Source: CAD feature listing. Evaluate the final solid. Frame: model axes, mm. Face numbers are marked on the shaded views. A direction names the side the tool comes from. Give positions to 0.01 mm unless a question says otherwise; leave off trailing zeros. Order: outer loops, then holes, each group sorted by start corner. A loop starts at its lowest first (then second) coordinate and runs counter-clockwise, first axis right, second up. Notation, with made-up numbers: (5.25, 23) - (11.25, 23) arc R19 ccw to (11.25, 32) - close; hole circle Ø11 at (39.5, 48.5). An arc over 180 degrees is marked (long way). Answer as CSV lines item,"result".
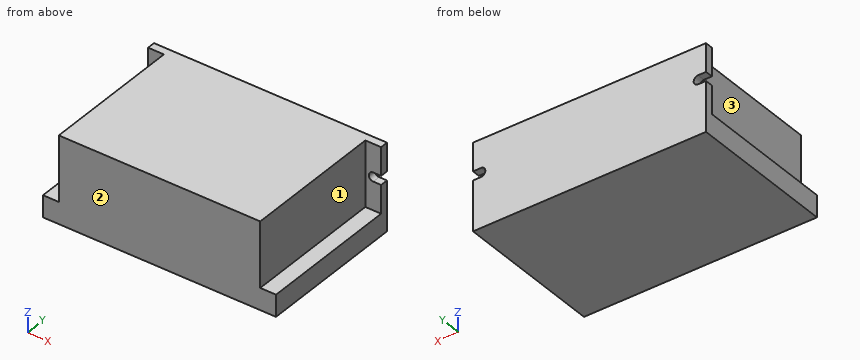
```python
from build123d import *

# Parameters (mm, degrees)
ESQUISSE1_W             = 118
ESQUISSE1_H             = 75.5
BOSS_EXTRU_1_DEPTH      = 11
BOSS_EXTRU_2_DEPTH      = 33
ENL_V_MAT_EXTRU_1_REACH = 107.929


with BuildPart() as part:
    # Esquisse1 → Boss.-Extru.1 (new body)
    with BuildSketch(Plane.XY):
        with Locations((-5.596837945, -6.384387352)):
            Rectangle(ESQUISSE1_W, ESQUISSE1_H)
    extrude(amount=BOSS_EXTRU_1_DEPTH)

    # Esquisse2 → Boss.-Extru.2 (add)
    with BuildSketch(Plane.XY.offset(11)):
        Polygon((-64.596837945, 31.365612648), (53.403162055, 31.365612648), (53.403162055, 27.365612648), (45.403162055, 27.365612648), (45.403162055, -44.134387352), (-56.596837945, -44.134387352), (-56.596837945, 27.365612648), (-64.596837945, 27.365612648), align=None)
    extrude(amount=BOSS_EXTRU_2_DEPTH)

    # Esquisse3 → Enlèv. mat.-Extru.1 (cut, up to next)
    with BuildSketch(Plane.XZ.offset(-27.365612648), mode=Mode.PRIVATE) as enl_v_mat_extru_1_sk1:
        with BuildLine():
            Line((-64.596837945, 29.75), (-60.596837945, 29.75))
            ThreePointArc((-60.596837945, 29.75), (-58.346837945, 27.5), (-60.596837945, 25.25))
            Line((-60.596837945, 25.25), (-64.596837945, 25.25))
            Line((-64.596837945, 25.25), (-64.596837945, 29.75))
        make_face()
    enl_v_mat_extru_1_tool1 = extrude(enl_v_mat_extru_1_sk1.sketch, amount=-ENL_V_MAT_EXTRU_1_REACH, mode=Mode.PRIVATE) & part.part
    # Esquisse3 → Enlèv. mat.-Extru.1 (cut, up to next)
    with BuildSketch(Plane.XZ.offset(-27.365612648), mode=Mode.PRIVATE) as enl_v_mat_extru_1_sk2:
        with BuildLine():
            Line((53.403162055, 29.75), (49.403162055, 29.75))
            ThreePointArc((49.403162055, 29.75), (47.153162055, 27.5), (49.403162055, 25.25))
            Line((49.403162055, 25.25), (53.403162055, 25.25))
            Line((53.403162055, 25.25), (53.403162055, 29.75))
        make_face()
    enl_v_mat_extru_1_tool2 = extrude(enl_v_mat_extru_1_sk2.sketch, amount=-ENL_V_MAT_EXTRU_1_REACH, mode=Mode.PRIVATE) & part.part
    add(enl_v_mat_extru_1_tool1.solids().sort_by_distance((-61.6914, 27.365613, 27.5))[0], mode=Mode.SUBTRACT)
    add(enl_v_mat_extru_1_tool2.solids().sort_by_distance((50.497724, 27.365613, 27.5))[0], mode=Mode.SUBTRACT)


solid = part.part
```
(1) Cut plane B-B (y = -37.5). Return loops of the section in (x, z).
Completed:
outline,"(-64.6, 0) - (53.4, 0) - (53.4, 11) - (45.4, 11) - (45.4, 44) - (-56.6, 44) - (-56.6, 11) - (-64.6, 11) - close"
(2) Cut plane A-A (z = 27.5). Return loops of the section in (x, y), then the cut area to 4 significant figures.
Completed:
outline,"(-58.35, 27.37) - (-56.6, 27.37) - (-56.6, -44.13) - (45.4, -44.13) - (45.4, 27.37) - (47.15, 27.37) - (47.15, 31.37) - (-58.35, 31.37) - close"
area,"7,715 mm²"
(3) Ray query, line 1 (Y direction, x = -58, z = 16.5); line 2 (X direction, y = -27.5, z = 40.5); line 3 (Z direction, x = 46.5, y = -33). Return the intervals inside material, ascending. Write a range as from..to.
Completed:
line 1,"27.37..31.37"
line 2,"-56.6..45.4"
line 3,"0..11"
(4) Contact query for flat-ended pins moving along their axis: pin 1 (2 mm diameter, centred on y = -15, z = 19.5, fed in from +X); pin 2 (8 mm diameter, centred on y = 9.5, z = 25, fed in from -X); pin 3 (9 mm diameter, centred on x = -62, z = 31.5, fed in from -Y). Output: stop coordinate, or through.
Completed:
pin 1,"x = 45.4"
pin 2,"x = -56.6"
pin 3,"y = 27.37"
(5) Access query for the marked faces 1, 2 and 3. Directions: +Z, -Z, +X, -X, +Y, -Y. A direction counts if a zero-diameter tool reaches every point of the face in a straight line with its end or side. Return the directions, or none.
Completed:
face 1,"+Z, +X, -Y"
face 2,"+Z, -Z, +X, -X, -Y"
face 3,"+Z, -X, -Y"
